```python
from build123d import *

# Parameters (mm, degrees)
SKETCH_1_W          = 48
SKETCH_1_H          = 15
SKETCH_1_R          = 1.1
SKETCH_1_R_2        = 1.5
SKETCH_1_R_3        = 2.5
EXTRUDE_1_DEPTH     = 2
EXTRUDE_2_DEPTH     = 2
SKETCH_4_R          = 3
CUT_EXTRUDE_1_DEPTH = 1.5
SKETCH_5_W          = 46
SKETCH_5_H          = 1.5
EXTRUDE_3_DEPTH     = 5
SKETCH_2_3_R        = 0.95
CUT_EXTRUDE_2_DEPTH = 6
CUT_EXTRUDE_START   = -0.25
SKETCH_7_R          = 0.95
CUT_EXTRUDE_3_DEPTH = 0.25
SKETCH_1_3_W        = 15
SKETCH_1_3_H        = 15
SKETCH_1_3_R        = 6
SKETCH_1_3_R_2      = 1.5
SKETCH_1_3_R_3      = 1.1
EXTRUDE_4_DEPTH     = 2
EXTRUDE_START       = -2
SKETCH_1_4_W        = 15
SKETCH_1_4_H        = 15
SKETCH_1_4_R        = 6
SKETCH_1_4_R_2      = 1.5
SKETCH_1_4_R_3      = 1.1
EXTRUDE_5_DEPTH     = 2
SKETCH_1_5_R        = 6
CUT_EXTRUDE_4_DEPTH = 2
CUT_EXTRUDE_5_DEPTH = 15


with BuildPart() as part:
    # 草图1 → 凸台-拉伸1 (new body)
    with BuildSketch(Plane(origin=(0, 0, 0), x_dir=(1, 0, 0), z_dir=(0, 1, 0))):
        with Locations((-7.5, 0)):
            Rectangle(SKETCH_1_W, SKETCH_1_H)
        with Locations(Location((-4.169872981, -2.5, 0), (0, 0, 270))):
            Circle(SKETCH_1_R, mode=Mode.SUBTRACT)
        with Locations(Location((3, 0, 0), (0, 0, 270))):
            Circle(SKETCH_1_R, mode=Mode.SUBTRACT)
        with Locations(Location((-8.5, 0, 0), (0, 0, 270))):
            Circle(SKETCH_1_R_2, mode=Mode.SUBTRACT)
        with Locations(Location((-12.830127019, 2.5, 0), (0, 0, 270))):
            Circle(SKETCH_1_R, mode=Mode.SUBTRACT)
        with Locations(Location((8, 0, 0), (0, 0, 270))):
            Circle(SKETCH_1_R_3, mode=Mode.SUBTRACT)
        with Locations(Location((13, 0, 0), (0, 0, 270))):
            Circle(SKETCH_1_R, mode=Mode.SUBTRACT)
        with Locations(Location((8, 5, 0), (0, 0, 270))):
            Circle(SKETCH_1_R, mode=Mode.SUBTRACT)
    extrude(amount=EXTRUDE_1_DEPTH)

    # 草图2 → 凸台-拉伸2 (add)
    with BuildSketch(Plane.XY.offset(7.5)):
        with BuildLine():
            Line((-22.1, 1.4), (-24.9, 1.4))
            ThreePointArc((-24.9, 1.4), (-23.5, 0), (-22.1, 1.4))
        make_face()
        with BuildLine():
            ThreePointArc((-24.764911064, 2), (-24.865810289, 1.707509764), (-24.9, 1.4))
            Line((-24.9, 1.4), (-22.1, 1.4))
            ThreePointArc((-22.1, 1.4), (-22.134189711, 1.707509764), (-22.235088936, 2))
            Line((-22.235088936, 2), (-24.764911064, 2))
        make_face()
        with BuildLine():
            ThreePointArc((-22.235088936, 2), (-23.5, 2.8), (-24.764911064, 2))
            Line((-24.764911064, 2), (-22.235088936, 2))
        make_face()
        with BuildLine():
            Line((-7.1, 1.4), (-9.9, 1.4))
            ThreePointArc((-9.9, 1.4), (-8.5, 0), (-7.1, 1.4))
        make_face()
        with BuildLine():
            ThreePointArc((-9.764911064, 2), (-9.865810289, 1.707509764), (-9.9, 1.4))
            Line((-9.9, 1.4), (-7.1, 1.4))
            ThreePointArc((-7.1, 1.4), (-7.134189711, 1.707509764), (-7.235088936, 2))
            Line((-7.235088936, 2), (-9.764911064, 2))
        make_face()
        with BuildLine():
            ThreePointArc((-7.235088936, 2), (-8.5, 2.8), (-9.764911064, 2))
            Line((-9.764911064, 2), (-7.235088936, 2))
        make_face()
        with BuildLine():
            Line((7.9, 1.4), (5.1, 1.4))
            ThreePointArc((5.1, 1.4), (6.5, 0), (7.9, 1.4))
        make_face()
        with BuildLine():
            ThreePointArc((5.235088936, 2), (5.134189711, 1.707509764), (5.1, 1.4))
            Line((5.1, 1.4), (7.9, 1.4))
            ThreePointArc((7.9, 1.4), (7.865810289, 1.707509764), (7.764911064, 2))
            Line((7.764911064, 2), (5.235088936, 2))
        make_face()
        with BuildLine():
            ThreePointArc((7.764911064, 2), (6.5, 2.8), (5.235088936, 2))
            Line((5.235088936, 2), (7.764911064, 2))
        make_face()
    extrude(amount=EXTRUDE_2_DEPTH)

    # 草图4 → 切除-拉伸1 (cut)
    with BuildSketch(Plane(origin=(0, 2, 0), x_dir=(1, 0, 0), z_dir=(0, 1, 0))):
        with Locations(Location((-8.5, 0, 0), (0, 0, 270))):
            Circle(SKETCH_4_R)
    extrude(amount=-CUT_EXTRUDE_1_DEPTH, mode=Mode.SUBTRACT)

    # 草图5 → 凸台-拉伸3 (add)
    with BuildSketch(Plane(origin=(0, 2, 0), x_dir=(1, 0, 0), z_dir=(0, 1, 0))):
        with Locations((-8.5, -6.75)):
            Rectangle(SKETCH_5_W, SKETCH_5_H)
    extrude(amount=EXTRUDE_3_DEPTH)

    # 草图2<3> → 切除-拉伸2 (cut)
    with BuildSketch(Plane.XY.offset(7.5)):
        with Locations((-23.5, 5.4)):
            Circle(SKETCH_2_3_R)
        with Locations((-8.5, 5.4)):
            Circle(SKETCH_2_3_R)
        with Locations((6.5, 5.4)):
            Circle(SKETCH_2_3_R)
    extrude(amount=-CUT_EXTRUDE_2_DEPTH, mode=Mode.SUBTRACT)

    # 草图7 → 切除-拉伸3 (cut)
    # profile 1 of 3: a face of its own
    with BuildSketch(Plane(origin=(0, 0, 6), x_dir=(-1, 0, 0), z_dir=(0, 0, -1)).offset(CUT_EXTRUDE_START)):
        Polygon((-7.596965511, 3.5), (-5.403034489, 3.5), (-4.306068977, 5.4), (-5.403034489, 7.3), (-7.596965511, 7.3), (-8.693931023, 5.4), align=None)
        with Locations(Location((-6.5, 5.4, 0), (0, 0, 180))):
            Circle(SKETCH_7_R, mode=Mode.SUBTRACT)
    # profile 2 of 3: a face of its own
    with BuildSketch(Plane(origin=(0, 0, 6), x_dir=(-1, 0, 0), z_dir=(0, 0, -1)).offset(CUT_EXTRUDE_START)):
        Polygon((6.306068977, 5.4), (7.403034489, 3.5), (9.596965511, 3.5), (10.693931023, 5.4), (9.596965511, 7.3), (7.403034489, 7.3), align=None)
        with Locations(Location((8.5, 5.4, 0), (0, 0, 180))):
            Circle(SKETCH_7_R, mode=Mode.SUBTRACT)
    # profile 3 of 3: a face of its own
    with BuildSketch(Plane(origin=(0, 0, 6), x_dir=(-1, 0, 0), z_dir=(0, 0, -1)).offset(CUT_EXTRUDE_START)):
        Polygon((21.306068977, 5.4), (22.403034489, 3.5), (24.596965511, 3.5), (25.693931023, 5.4), (24.596965511, 7.3), (22.403034489, 7.3), align=None)
    extrude(amount=CUT_EXTRUDE_3_DEPTH, mode=Mode.SUBTRACT)

    # 草图1<3> → 凸台-拉伸4 (add)
    # profile 1 of 2: a face of its own
    with BuildSketch(Plane(origin=(0, 0, 0), x_dir=(1, 0, 0), z_dir=(0, 1, 0))):
        with Locations((24, 0)):
            Rectangle(SKETCH_1_3_W, SKETCH_1_3_H)
        with Locations((24, 0)):
            Circle(SKETCH_1_3_R, mode=Mode.SUBTRACT)
    # profile 2 of 2: a face of its own
    with BuildSketch(Plane(origin=(0, 0, 0), x_dir=(1, 0, 0), z_dir=(0, 1, 0))):
        with Locations((24, 0)):
            Circle(SKETCH_1_3_R)
        with Locations(Location((24, 0, 0), (0, 0, 270))):
            Circle(SKETCH_1_3_R_2, mode=Mode.SUBTRACT)
        with Locations(Location((27.5, 0, 0), (0, 0, 270))):
            Circle(SKETCH_1_3_R_3, mode=Mode.SUBTRACT)
        with Locations(Location((24, -3.5, 0), (0, 0, 270))):
            Circle(SKETCH_1_3_R_3, mode=Mode.SUBTRACT)
        with Locations(Location((20.5, 0, 0), (0, 0, 270))):
            Circle(SKETCH_1_3_R_3, mode=Mode.SUBTRACT)
        with Locations(Location((24, 3.5, 0), (0, 0, 270))):
            Circle(SKETCH_1_3_R_3, mode=Mode.SUBTRACT)
    extrude(amount=EXTRUDE_4_DEPTH)

    # 草图1<4> → 凸台-拉伸5 (add)
    # profile 1 of 2: a face of its own
    with BuildSketch(Plane(origin=(0, 0, 0), x_dir=(1, 0, 0), z_dir=(0, 1, 0)).offset(EXTRUDE_START)):
        with Locations((24, 0)):
            Rectangle(SKETCH_1_4_W, SKETCH_1_4_H)
        with Locations((24, 0)):
            Circle(SKETCH_1_4_R, mode=Mode.SUBTRACT)
    # profile 2 of 2: a face of its own
    with BuildSketch(Plane(origin=(0, 0, 0), x_dir=(1, 0, 0), z_dir=(0, 1, 0)).offset(EXTRUDE_START)):
        with Locations((24, 0)):
            Circle(SKETCH_1_4_R)
        with Locations(Location((24, 0, 0), (0, 0, 270))):
            Circle(SKETCH_1_4_R_2, mode=Mode.SUBTRACT)
        with Locations(Location((27.5, 0, 0), (0, 0, 270))):
            Circle(SKETCH_1_4_R_3, mode=Mode.SUBTRACT)
        with Locations(Location((24, -3.5, 0), (0, 0, 270))):
            Circle(SKETCH_1_4_R_3, mode=Mode.SUBTRACT)
        with Locations(Location((20.5, 0, 0), (0, 0, 270))):
            Circle(SKETCH_1_4_R_3, mode=Mode.SUBTRACT)
        with Locations(Location((24, 3.5, 0), (0, 0, 270))):
            Circle(SKETCH_1_4_R_3, mode=Mode.SUBTRACT)
    extrude(amount=EXTRUDE_5_DEPTH)

    # 草图1<5> → 切除-拉伸4 (cut)
    with BuildSketch(Plane(origin=(0, 0, 0), x_dir=(1, 0, 0), z_dir=(0, 1, 0))):
        with Locations(Location((24, 0, 0), (0, 0, 270))):
            Circle(SKETCH_1_5_R)
    extrude(amount=CUT_EXTRUDE_4_DEPTH, mode=Mode.SUBTRACT)

    # 草图8 → 切除-拉伸5 (cut)
    with BuildSketch(Plane(origin=(0, 0, -7.5), x_dir=(-1, 0, 0), z_dir=(0, 0, -1))):
        Polygon((-16.5, 0), (-18.5, -2), (-16.5, -2), align=None)
    extrude(amount=-CUT_EXTRUDE_5_DEPTH, mode=Mode.SUBTRACT)


solid = part.part
```
Input: part model. Units: mm. Frame: model coordinates. A direction names the side the tool comes from. Round coordinates to 2 decimals unless told otherwise and drop trailing zeros. Loops run counter-clockwise (first coordinate to the right, second up) from the corner with the lowest first, then second, coordinate; pieces in that order, holes last. Notation, with made-up numbers: (-5.75, -16.75) - (36.25, -16.75) arc R24 ccw to (36.25, -6.75) - close; hole circle Ø8 at (76, 52.5). An arc over 180 degrees is marked (long way). One line per item, written item: value. Start each with the question number.
(1) Ray query, line 1 (X direction, y = 2, z = 8.5); line 2 (Z direction, x = 24, y = -0.95); line 3 (X direction, y = 1.2, z = 0). Return the intervals inside material, ascending. Write a range as [from, to].
(2) Contact query for flat-ended pins moving along their axis: P1, Ø5, axis at x = -9, z = 1.5, coming from the +Y side; P2, Ø1.6, axis at y = 5, z = 6.5, coming from the +X side; P3, Ø5, axis at x = -18.5, z = 2.5, coming from the -Y side. Output: stop coordinate, or through.
(3) Access query for faces 1 (the cylindrical face through (-5.526, 1.26, -0.391)), 2 (the flat face through (-8, 0, 2)), 3 (the flat face through (-24, 4, 6.25)). Directions: +Z, -Z, +X, -X, +Y, -Y. A direction counts if a zero-diameter tool reaches every point of the face in a straight line with its end or side. Return the directions, or none.
(4) Section B-B, the plane x = 3. Return loops of the section in (y, z), plus the area to 3 significant figures.
(5) Section A-A, the plane x = 24. Return loops of the section in (y, z), plus the area to 3 significant figures.
(6) Draft query along X for faces 4 (the cylindrical face through (26.426, -1.014, -0.238)), 5 (the cylindrical face through (3.93, 0.99, 0.59)), 6 (the flat face through (26, -2, 0)), 7 (the flat face through (31.5, 0, 0)). Return one class per face: +X half, -X half, draft (parallel to the pull), parting line (faces both ways), or undercut.
Results below:
1. line 1: [-24.76, -22.24], [-9.76, -7.24], [5.24, 7.76]
1. line 2: [-7.5, -4.6], [-2.4, -1.5], [1.5, 2.4], [4.6, 7.5]
1. line 3: [-31.5, -11.5], [-5.5, 1.9], [4.1, 5.5], [10.5, 11.9], [14.1, 18], [30, 31.5]
2. P1: y = 2
2. P2: x = 14.5
2. P3: y = 0
3. face 1: +Y
3. face 2: +Z, -Z, -X, -Y
3. face 3: -Z
4. outline: (0, -7.5) - (2, -7.5) - (2, -1.1) - (0, -1.1) - close; (0, 1.1) - (2, 1.1) - (2, 6) - (7, 6) - (7, 7.5) - (0, 7.5) - close
4. area: 33.1 mm^2
5. outline: (-2, -7.5) - (2, -7.5) - (2, -6) - (0, -6) - (0, -4.6) - (-2, -4.6) - close; (-2, -2.4) - (0, -2.4) - (0, -1.5) - (-2, -1.5) - close; (-2, 1.5) - (0, 1.5) - (0, 2.4) - (-2, 2.4) - close; (-2, 4.6) - (0, 4.6) - (0, 6) - (2, 6) - (2, 7.5) - (-2, 7.5) - close
5. area: 21.2 mm^2
6. face 4: undercut
6. face 5: undercut
6. face 6: draft
6. face 7: +X half
